Can you work these out from the model? Positions are in its coordinate system, mm. A direction names the side the tool comes from. Round coordinates to 2 decimals unless told otherwise and drop trailing zeros. Loops run counter-clockwise (first coordinate to the right, second up) from the corner with the lowest first, then second, coordinate; pieces in that order, holes last.
(1) I want a section at B-B on y = 2.5. Write out the boundary of the cut face in (x, z) (1 decimal), plus the area to 3 significant figures.
(2) Will these pins go through, and if not, where does the flat tip stop? pin 1 Ø3 at (x, y) = (-10, 15) entering from -Z; pin 2 Ø8 at (x, z) = (13, -14) entering from +Y; pin 3 Ø12 at (y, z) = (11, 20) entering from +X; pin 4 Ø11 at (y, z) = (21.5, 4) entering from +X.
(3) Which directions (+Z, -Z, +X, -X, +Y, -Y) give clear straight access to the entire face, cutting with the end or side of a thin tool? Please do faces 1 (the face through (19.05, 18, 0)), 2 (the face through (-19.05, 18, 0)), 3 (the face through (21, 3.175, 0)), 4 (the face through (17.13, 31.05, -9.83)), 5 (the face through (-9.9, 3.61, -16.81)).
(4) Thinking about a two-plate mould opening in X: for faces 6 (the face through (-9.392, 18.035, -16.575)), 7 (the face through (-10.6, 15.65, -3.34)), 8 (the face through (0, 31, 19.8)), 9 (the face through (9.61, 3.61, -16.98)), which applies, released by +X, released by -X, zero draft, split by the parting line, or undercut?
(5) If I drill on line 1 along Z through (x, y) = (0, 13); line 2 along Y through (x, z) = (-4, 22.5) (3 decimals); line 3 along X through (y, z) = (9, 5.5), over which ranges is the centre line in solid material (lowest first)?
from build123d import *

# Parameters (mm, degrees)
SKETCH2_R                = 25.4
BOSS_EXTRUDE1_DEPTH      = 3.175
BOSS_EXTRUDE2_DEPTH      = 28.575
F_1_8_TAPPED_HOLE1_D     = 22.225
F_1_8_TAPPED_HOLE1_DEPTH = 31.75
FILLET1_R                = 1.524


with BuildPart() as part:
    # Sketch2 → Boss-Extrude1 (new body)
    with BuildSketch(Plane(origin=(0, 0, 0), x_dir=(1, 0, 0), z_dir=(0, 1, 0))):
        Circle(SKETCH2_R)
    extrude(amount=BOSS_EXTRUDE1_DEPTH)

    # Sketch3 → Boss-Extrude2 (add)
    with BuildSketch(Plane(origin=(0, 3.175, 0), x_dir=(1, 0, 0), z_dir=(0, 1, 0))):
        Polygon((0, 21.997045256), (-19.05, 10.998522628), (-19.05, -10.998522628), (0, -21.997045256), (19.05, -10.998522628), (19.05, 10.998522628), align=None)
    extrude(amount=BOSS_EXTRUDE2_DEPTH)

    # 1-8 Tapped Hole1
    with Locations(Plane(origin=(0, 31.75, 0), x_dir=(1, 0, 0), z_dir=(0, 1, 0))):
        with Locations((0, 0)):
            Hole(F_1_8_TAPPED_HOLE1_D / 2, depth=F_1_8_TAPPED_HOLE1_DEPTH)

    # Cut-Sweep1: sweep along a path in Sketch7
    with BuildLine(Plane(origin=(0, 31.75, 0), x_dir=(1, 0, 0), z_dir=(0, 1, 0))) as cut_sweep1_path:
        CenterArc((0, 0), 19.05, 0, 360)
    # Sketch8 → Cut-Sweep1 (sweep, cut)
    with BuildSketch(Plane(origin=(0, 0, 0), x_dir=(0, 0, -1), z_dir=(1, 0, 0))):
        Polygon((-21.997045256, 28.802954744), (-21.997045256, 31.75), (-19.05, 31.75), align=None)
    sweep(path=cut_sweep1_path.line, mode=Mode.SUBTRACT)

    # Fillet1
    fillet1_edges = [part.edges().sort_by_distance(p)[0] for p in [
        (9.525, 3.175, -16.497783942),
        (-9.525, 3.175, -16.497783942),
        (-19.05, 3.175, 0),
        (-9.525, 3.175, 16.497783942),
        (9.525, 3.175, 16.497783942),
        (19.05, 3.175, 0),
    ]]
    fillet(fillet1_edges, radius=FILLET1_R)


solid = part.part
Filled sheet:
1. outline: circle Ø50.8 at (0, 0); hole circle Ø22.2 at (0, 0)
1. area: 1,640 mm2
2. pin 1: stops at z = -17.09
2. pin 2: stops at y = 31.75
2. pin 3: stops at x = 13.85
2. pin 4: stops at x = 19.05
3. face 1: +Z, -Z, +X, +Y
3. face 2: +Z, -Z, -X, +Y
3. face 3: +Y
3. face 4: -Z, +X, +Y
3. face 5: -Z, -X, +Y
4. face 6: released by -X
4. face 7: undercut
4. face 8: split by the parting line
4. face 9: released by +X
5. line 1: z = -22 to -11.11, 11.11 to 22
5. line 2: y = 0 to 3.175
5. line 3: x = -19.05 to -9.66, 9.66 to 19.05
